```python
from build123d import *

# Parameters (mm, degrees)
SKETCH1_W           = 58
SKETCH1_H           = 35
SKETCH1_R           = 1
BOSS_EXTRUDE1_DEPTH = 2
SKETCH2_W           = 48
SKETCH2_H           = 35
BOSS_EXTRUDE2_DEPTH = 3


with BuildPart() as part:
    # Sketch1 → Boss-Extrude1 (new body)
    with BuildSketch(Plane.XY):
        with Locations((29, 17.5)):
            Rectangle(SKETCH1_W, SKETCH1_H)
        with Locations((2.5, 32.5)):
            Circle(SKETCH1_R, mode=Mode.SUBTRACT)
        with Locations(Location((55.5, 32.5, 0), (0, 0, 180))):
            Circle(SKETCH1_R, mode=Mode.SUBTRACT)
        with Locations(Location((2.5, 2.5, 0), (0, 0, 180))):
            Circle(SKETCH1_R, mode=Mode.SUBTRACT)
        with Locations((55.5, 2.5)):
            Circle(SKETCH1_R, mode=Mode.SUBTRACT)
    extrude(amount=BOSS_EXTRUDE1_DEPTH)

    # Sketch2 → Boss-Extrude2 (add)
    with BuildSketch(Plane.XY.offset(2)):
        with Locations((29, 17.5)):
            Rectangle(SKETCH2_W, SKETCH2_H)
    extrude(amount=BOSS_EXTRUDE2_DEPTH)


solid = part.part
```
Can you work these out from the model? Positions are in its coordinate system, mm. A direction names the side the tool comes from. Give positions to 0.01 mm unless a question says otherwise; leave off trailing zeros. Order: outer loops, then holes, each group sorted by start corner. A loop starts at its lowest first (then second) coordinate and runs counter-clockwise, first axis right, second up. Notation, with made-up numbers: M -40,34 L -16,34 A35 ccw -16,73 Z; hole C 89,35 d1. An arc over 180 degrees is marked long. Write item = value, one per line. Start each with the question number.
Q1. Will these pins go through, and if not, where does the flat tip stop? pin 1 Ø1.2 at (x, y) = (55.5, 2.5) entering from +Z; pin 2 Ø2 at (y, z) = (22, 3.5) entering from -X; pin 3 Ø2.5 at (x, y) = (55.5, 32.5) entering from +Z.
Q2. We'd pull the mould along X, two halves only. Please class faces 4 (the flat face through (0, 17, 1)), 5 (the cylindrical face through (2.37, 33.49, 0.99)), 6 (the flat face through (2, 18, 2)), 7 (the flat face through (58, 17, 1)): pulls with the +X half, pulls with the -X half, needs draft (parallel to the pull), parting line crosses it, or undercut.
Q3. Suppose I cut it at B-B (x = 2.5). Write out the boundary of the cut face in (y, z), plus the area to 3 significant figures.
Q4. Suppose I cut it at C-C (y = 14.5). Write out the boundary of the cut face in (x, z).
Q5. For faces 1 (the flat face through (5, 17, 3)), 2 (the flat face through (29, 0, 2)), 3 (the flat face through (55, 18, 2)), which set-ups out of +Z, -Z, +X, -X, +Y, -Y let a thin tool reach every point of the face, with its end or its side?
Q6. Suppose I cut it at D-D (z = 2.8). Write out the boundary of the cut face in (x, y).
Q7. I need wall thicknesses on probe 1 along Y at (x, z) = (2.5, 0.5); probe 2 along X at (y, z) = (12, 4.5). Which ranges of each line are inside material? Lowest first, please. Write a range as [from, to].
Q8. Suppose I cut it at A-A (y = 32.5). Write out the boundary of the cut face in (x, z).
Check result:
q1.pin_1 = through
q1.pin_2 = 5
q1.pin_3 = 2
q2.face_4 = pulls with the -X half
q2.face_5 = undercut
q2.face_6 = needs draft
q2.face_7 = pulls with the +X half
q3.outline = M 0,0 L 1.5,0 L 1.5,2 L 0,2 Z; M 3.5,0 L 31.5,0 L 31.5,2 L 3.5,2 Z; M 33.5,0 L 35,0 L 35,2 L 33.5,2 Z
q3.area = 62.0 mm2
q4.outline = M 0,0 L 58,0 L 58,2 L 53,2 L 53,5 L 5,5 L 5,2 L 0,2 Z
q5.face_1 = +Z, -X, +Y, -Y
q5.face_2 = +Z, -Z, +X, -X, -Y
q5.face_3 = +Z, +X, +Y, -Y
q6.outline = M 5,0 L 53,0 L 53,35 L 5,35 Z
q7.probe_1 = [0, 1.5], [3.5, 31.5], [33.5, 35]
q7.probe_2 = [5, 53]
q8.outline = M 0,0 L 1.5,0 L 1.5,2 L 0,2 Z; M 3.5,0 L 54.5,0 L 54.5,2 L 53,2 L 53,5 L 5,5 L 5,2 L 3.5,2 Z; M 56.5,0 L 58,0 L 58,2 L 56.5,2 Z
